Study the drawing (mm; zero at the part's minimum x, y, z) and answer. Coordinates: 2 decimals unless noted, no trailing zeros. Order: outer loops, then holes, each group sorted by start corner. A loop starts at its lowest first (then second) coordinate and runs counter-clockwise, first axis right, second up. Notation, with made-up numbers: (2, -22.75) -> (46, -22.75) arc R20 cw to (46, -7.75) -> close; hole circle Ø6 at (-24, 43). An arc over 180 degrees is marked (long way). Write each question's results on one line, items separated by ' | '. Start each with the question number.
(1) The part is cut by section A-A, the plane y = 65. Give the vertices of the cut face in (x, z).
(2) The part is cut by section D-D, the plane y = 5. Give the vertices of the cut face in (x, z).
(3) Straight lines are drawn through the part: L1, parallel to Y at x = 49, z = 2.65; L2, parallel to X at y = 65, z = 1.9; L3, parallel to Y at x = 48, z = 2.55. For each, find the intervals that lie inside material, in ascending order.
(4) Given pin 1 (2 mm diameter, centred on y = 27, z = 0.5, fed in from +X), flat-ended and moving along its own axis, determine where the tip first touches the part or whether it passes through.
(5) The part is cut by section C-C, the plane x = 49. Give the vertices of the cut face in (y, z), then the cut area to 3 significant figures.
(6) The part is cut by section B-B, the plane z = 1.85. Give the vertices of the cut face in (x, y).
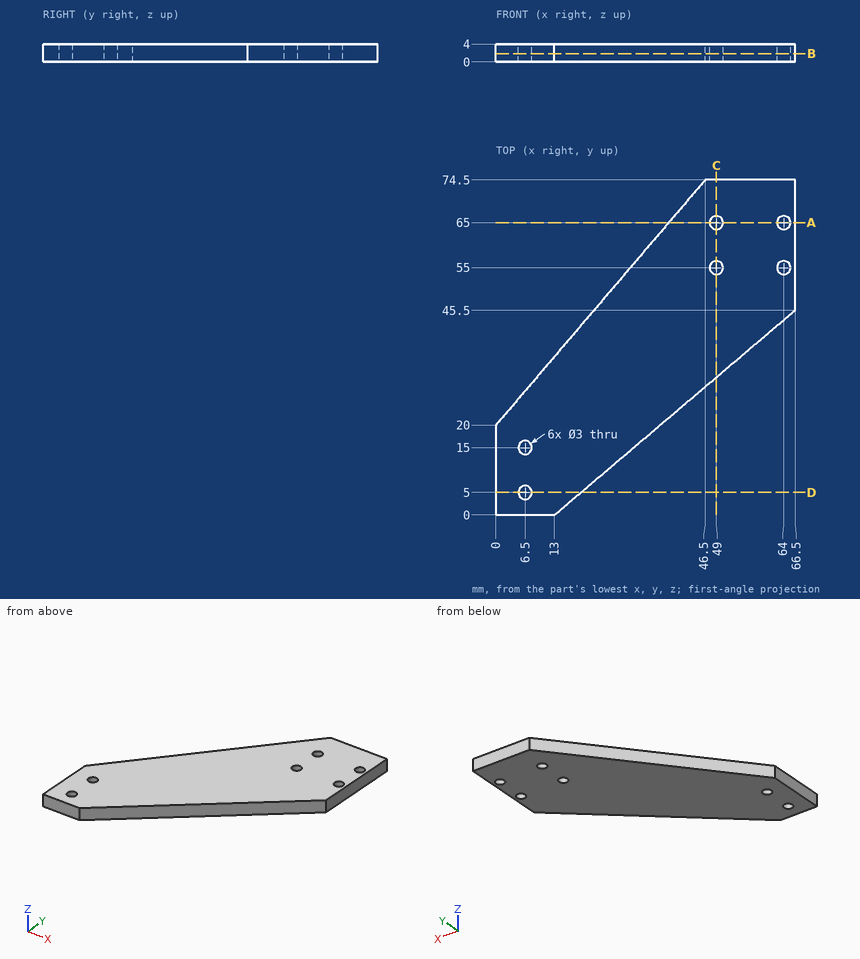
Established:
1) outline: (38.39, 0) -> (47.5, 0) -> (47.5, 4) -> (38.39, 4) -> close; (50.5, 0) -> (62.5, 0) -> (62.5, 4) -> (50.5, 4) -> close; (65.5, 0) -> (66.5, 0) -> (66.5, 4) -> (65.5, 4) -> close
2) outline: (0, 0) -> (5, 0) -> (5, 4) -> (0, 4) -> close; (8, 0) -> (18.88, 0) -> (18.88, 4) -> (8, 4) -> close
3) L1: y = 30.62 to 53.5, 56.5 to 63.5, 66.5 to 74.5 | L2: x = 38.39 to 47.5, 50.5 to 62.5, 65.5 to 66.5 | L3: y = 29.77 to 53.88, 56.12 to 63.88, 66.12 to 74.5
4) pin 1: stops at x = 45.92
5) outline: (30.62, 0) -> (53.5, 0) -> (53.5, 4) -> (30.62, 4) -> close; (56.5, 0) -> (63.5, 0) -> (63.5, 4) -> (56.5, 4) -> close; (66.5, 0) -> (74.5, 0) -> (74.5, 4) -> (66.5, 4) -> close | area: 152 mm^2
6) outline: (0, 0) -> (13, 0) -> (66.5, 45.5) -> (66.5, 74.5) -> (46.5, 74.5) -> (0, 20) -> close; hole circle Ø3 at (6.5, 5); hole circle Ø3 at (6.5, 15); hole circle Ø3 at (49, 55); hole circle Ø3 at (49, 65); hole circle Ø3 at (64, 55); hole circle Ø3 at (64, 65)
